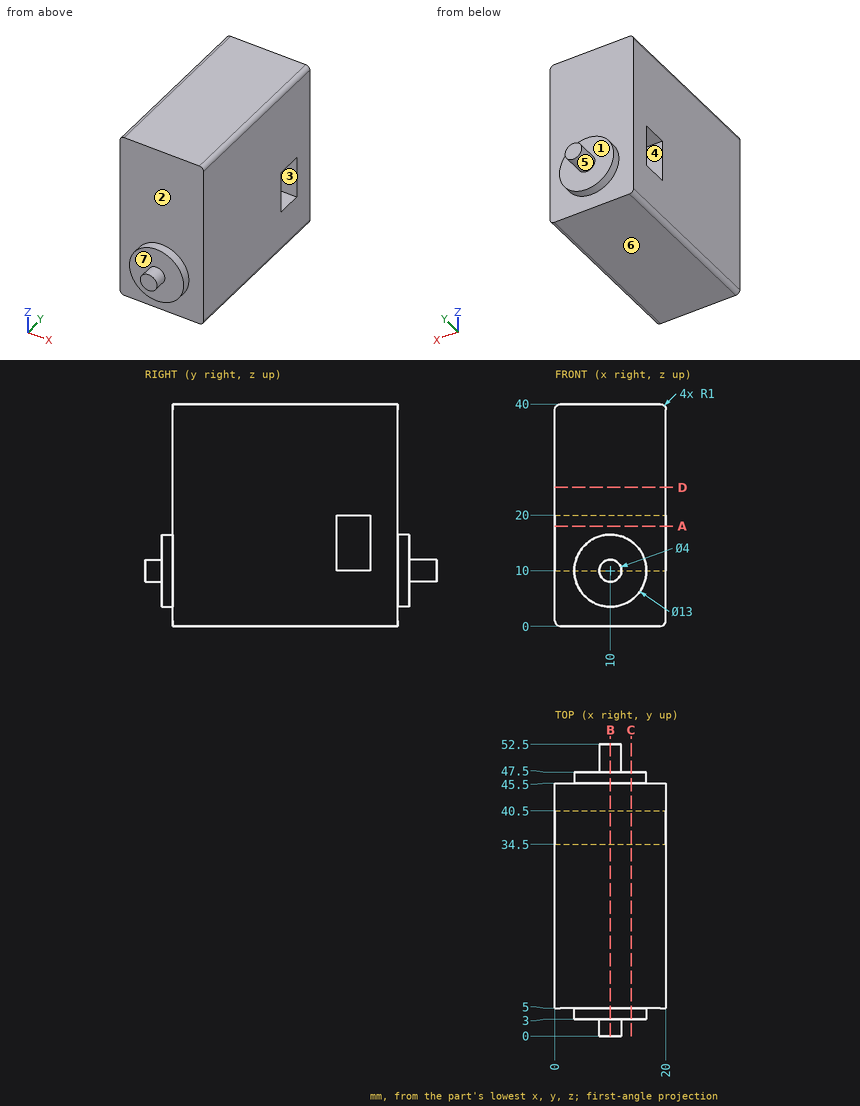
Print and shaded views of the part. All mm, measured from the part's lowest x, y and z. A direction names the side the tool comes from. Give positions to 0.01 mm unless a question says otherwise; leave off trailing zeros. Loops run counter-clockwise (first coordinate to the right, second up) from the corner with the lowest first, then second, coordinate; pieces in that order, holes last. Notation, with made-up numbers: (-28, 84) - (4, 84) arc R8 cw to (4, 88) - close; hole circle Ø3 at (18, 60). An arc over 180 degrees is marked (long way). One line per item, written item: value. Start each with the question number.
1. Slice it at B-B (x = 10). List the corners of the cut face in (y, z), plus the area to 3 significant figures.
2. Pin check, flat tips, straight feed: pin 1 (8 mm diameter, centred on x = 8, z = 23.5, fed in from +Y); pin 2 (8 mm diameter, centred on x = 12.5, z = 30.5, fed in from -Y); pin 3 (3 mm diameter, centred on x = 6.5, z = 13.5, fed in from -Y). Stop position of each tip, or through.
3. Slice it at A-A (z = 18). List the corners of the cut face in (x, y), plus the area to 3 significant figures.
4. Which spindle directions (+Z, -Z, +X, -X, +Y, -Y) get a long thin tool onto all of the face, cutting with end or side? Do the marked faces 5, 6 and 7. Say none if no direction does.
5. Slice it at D-D (z = 25). List the corners of the cut face in (x, y).
6. Slice it at C-C (x = 13.75). List the corners of the cut face in (y, z), plus the area to 3 significant figures.
7. Probe L1, parallel to Y at x = 2.5, z = 10.5; L2, parallel to Z at x = 17.5, y = 35; L3, parallel to Y at x = 7.5, z = 29.5. List the from-to ranges inside material, lowest first. Write a range as from..to.
8. Pull direction Y, two halves, no side cores. Call the marked faces 1, 2, 3 and 4: pulls with the +Y half, pulls with the -Y half, needs draft (parallel to the pull), parting line crosses it, or undercut.
Solution:
1. outline: (0, 8) - (3, 8) - (3, 3.5) - (5, 3.5) - (5, 0) - (45.5, 0) - (45.5, 3.5) - (47.5, 3.5) - (47.5, 8) - (52.5, 8) - (52.5, 12) - (47.5, 12) - (47.5, 16.5) - (45.5, 16.5) - (45.5, 40) - (5, 40) - (5, 16.5) - (3, 16.5) - (3, 12) - (0, 12) - close; hole (34.5, 10) - (40.5, 10) - (40.5, 20) - (34.5, 20) - close
1. area: 1,640 mm^2
2. pin 1: stops at y = 45.5
2. pin 2: stops at y = 5
2. pin 3: stops at y = 3
3. outline: (0, 5) - (20, 5) - (20, 34.5) - (0, 34.5) - close; (0, 40.5) - (20, 40.5) - (20, 45.5) - (0, 45.5) - close
3. area: 690 mm^2
4. face 5: +Y
4. face 6: -Z, +X, -X, +Y, -Y
4. face 7: -Y
5. outline: (0, 5) - (20, 5) - (20, 45.5) - (0, 45.5) - close
6. outline: (3, 4.69) - (5, 4.69) - (5, 0) - (45.5, 0) - (45.5, 4.69) - (47.5, 4.69) - (47.5, 15.31) - (45.5, 15.31) - (45.5, 40) - (5, 40) - (5, 15.31) - (3, 15.31) - close; hole (34.5, 10) - (40.5, 10) - (40.5, 20) - (34.5, 20) - close
6. area: 1,600 mm^2
7. L1: y = 5..34.5, 40.5..45.5
7. L2: z = 0..10, 20..40
7. L3: y = 5..45.5
8. face 1: pulls with the +Y half
8. face 2: pulls with the -Y half
8. face 3: undercut
8. face 4: undercut
